Part model, mm, in its own coordinate system. A direction names the side the tool comes from. Give positions to 0.01 mm unless a question says otherwise; leave off trailing zeros. Loops run counter-clockwise (first coordinate to the right, second up) from the corner with the lowest first, then second, coordinate; pieces in that order, holes last. Notation, with made-up numbers: (-7.75, 14) -> (9.25, 14) arc R24 cw to (9.25, 38) -> close; hole circle Ø10 at (67, 36). An arc over 180 degrees is marked (long way). One line per question, with ' | ' between items.
```python
from build123d import *

# Parameters (mm, degrees)
F1_DEPTH = 0.5
F3_DEPTH = 0.5
F4_R     = 10
F5_DEPTH = 1.001


with BuildPart() as f1:
    # F0 (on Top) → F1 (new body)
    with BuildSketch(Plane.XY):
        Polygon((0, 0), (-590, 0), (-622.5, -100), (-567.5, -480), (-22.5, -480), (32.5, -100), align=None)
    extrude(amount=F1_DEPTH)

    # F2 (on face) → F3 (join)
    with BuildSketch(Plane.XY.offset(0.5)):
        Polygon((0, 0), (-590, 0), (-560, -60), (-30, -60), align=None)
        Polygon((-567.5, -480), (-22.5, -480), (-30, -420), (-560, -420), align=None)
    extrude(amount=F3_DEPTH)

    # F4 (on face) → F5 (cut, through all)
    with BuildSketch(Plane.XY.offset(1)):
        with Locations((-500, -30)):
            Circle(F4_R)
        with Locations((-500, -450)):
            Circle(F4_R)
        with Locations((-90, -30)):
            Circle(F4_R)
        with Locations((-90, -450)):
            Circle(F4_R)
    extrude(amount=-F5_DEPTH, mode=Mode.SUBTRACT)


solid = f1.part
```
1) Tool access for faces 1 (the cylindrical face through (-490.46, -27, 0.51)), 2 (the flat face through (-575.2, -29.6, 0.7)): list every direction of +Z, -Z, +X, -X, +Y, -Y with a clear straight run to the whole face (end or side of a thin tool).
Found:
face 1: +Z, -Z | face 2: +Z, -X
2) Saw through at D-D (x = -170.5). Give the cut face in (y, z), and give its area (3 significant figures).
Found:
outline: (-480, 0) -> (0, 0) -> (0, 1) -> (-60, 1) -> (-60, 0.5) -> (-420, 0.5) -> (-420, 1) -> (-480, 1) -> close | area: 300 mm2
3) Saw through at C-C (y = -450). Give the cut face in (x, z).
Found:
outline: (-571.84, 0) -> (-510, 0) -> (-510, 1) -> (-563.75, 1) -> (-563.75, 0.5) -> (-571.84, 0.5) -> close; (-490, 0) -> (-100, 0) -> (-100, 1) -> (-490, 1) -> close; (-80, 0) -> (-18.16, 0) -> (-18.16, 0.5) -> (-26.25, 0.5) -> (-26.25, 1) -> (-80, 1) -> close
4) Saw through at A-A (z = 0.65). Give the cut face in (x, y).
Found:
outline: (-590, 0) -> (-560, -60) -> (-30, -60) -> (0, 0) -> close; (-567.5, -480) -> (-22.5, -480) -> (-30, -420) -> (-560, -420) -> close; hole circle Ø20 at (-500, -450); hole circle Ø20 at (-500, -30); hole circle Ø20 at (-90, -450); hole circle Ø20 at (-90, -30)
5) Drill centre lines: line 1 (Y direction, x = -500, z = 0.75); line 2 (Y direction, x = -221, z = 0.8); line 3 (Z direction, x = -432, y = -366). Where is each one in solid material? Low to high.
Found:
line 1: -480 to -460, -440 to -420, -60 to -40, -20 to 0 | line 2: -480 to -420, -60 to 0 | line 3: 0 to 0.5
6) Saw through at B-B (x = -500). Give the cut face in (y, z).
Found:
outline: (-480, 0) -> (-460, 0) -> (-460, 1) -> (-480, 1) -> close; (-440, 0) -> (-40, 0) -> (-40, 1) -> (-60, 1) -> (-60, 0.5) -> (-420, 0.5) -> (-420, 1) -> (-440, 1) -> close; (-20, 0) -> (0, 0) -> (0, 1) -> (-20, 1) -> close
7) Pin check, flat tips, straight feed: P1, Ø16, axis at x = -90, y = -30, coming from the -Z side; P2, Ø5, axis at x = -490, y = -225.5, coming from the +Z side; P3, Ø0.6, axis at x = -417, z = 0.5, coming from the +Y side. Stop position of each tip, or through.
Found:
P1: through | P2: z = 0.5 | P3: y = 0
8) Pull direction X, two halves, no side cores. Call faces 3 (the cylindrical face through (-490.46, -447, 0.51)), 4 (the flat face through (-300, -237, 0.5)), 5 (the flat face through (-15.2, -30.4, 0.7)): pulls with the +X half, pulls with the -X half, needs draft (parallel to the pull), parting line crosses it, or undercut.
Found:
face 3: undercut | face 4: needs draft | face 5: pulls with the +X half
